Here's how the part is built. I have some questions about the finished solid (model axes, mm). A direction names the side the tool comes from. Round coordinates to 2 decimals unless told otherwise and drop trailing zeros. Loops run counter-clockwise (first coordinate to the right, second up) from the corner with the lowest first, then second, coordinate; pieces in that order, holes last. Notation, with made-up numbers: M 12.5,5.5 L 67.5,5.5 A23 cw 67.5,27.5 Z; hole C 70,-23.75 d1. An arc over 180 degrees is marked long. Write each question's results on one line, items separated by ' | '. Start each with the question number.
```python
from build123d import *

# Parameters (mm, degrees)
SKETCH_1_W          = 15
SKETCH_1_H          = 26
SKETCH_1_R          = 2.5
SKETCH_1_R_2        = 1.5
EXTRUDE_1_DEPTH     = 4
SKETCH_14_W         = 15
SKETCH_14_H         = 6
EXTRUDE_4_DEPTH     = 20
EXTRUDE_5_DEPTH     = 4
SKETCH_17_W         = 40
SKETCH_17_H         = 10
CUT_EXTRUDE_3_DEPTH = 1.5
SKETCH_18_R         = 1.5
CUT_EXTRUDE_4_DEPTH = 2.5
CUT_EXTRUDE_5_DEPTH = 1.5
SKETCH_20_R         = 1.5
CUT_EXTRUDE_6_DEPTH = 2.5
FILLET_1_R          = 2
FILLET_2_R          = 1


with BuildPart() as part:
    # 草图1 → 凸台-拉伸1 (new body)
    with BuildSketch(Plane.XY):
        with Locations((0, -3)):
            Rectangle(SKETCH_1_W, SKETCH_1_H)
        Circle(SKETCH_1_R, mode=Mode.SUBTRACT)
        with Locations((-4, 6)):
            Circle(SKETCH_1_R_2, mode=Mode.SUBTRACT)
        with Locations((4, -6)):
            Circle(SKETCH_1_R_2, mode=Mode.SUBTRACT)
    extrude(amount=EXTRUDE_1_DEPTH)

    # 草图14 → 凸台-拉伸4 (add)
    with BuildSketch(Plane.XY.offset(4)):
        with Locations((0, -13)):
            Rectangle(SKETCH_14_W, SKETCH_14_H)
    extrude(amount=EXTRUDE_4_DEPTH)

    # 草图15 → 凸台-拉伸5 (add)
    with BuildSketch(Plane.XY.offset(24)):
        Polygon((-7.5, -10), (-7.5, -39.01879788), (-26.52, -50), (-77.5, -50), (-77.5, -65), (-22.5, -65), (7.5, -47.679491924), (7.5, -10), align=None)
    extrude(amount=EXTRUDE_5_DEPTH)

    # 草图17 → 切除-拉伸3 (cut)
    with BuildSketch(Plane(origin=(0, 0, 24), x_dir=(-1, 0, 0), z_dir=(0, 0, -1))):
        with Locations((54.5, -57.5)):
            Rectangle(SKETCH_17_W, SKETCH_17_H)
    extrude(amount=-CUT_EXTRUDE_3_DEPTH, mode=Mode.SUBTRACT)

    # 草图18 → 切除-拉伸4 (cut)
    with BuildSketch(Plane(origin=(0, 0, 25.5), x_dir=(-1, 0, 0), z_dir=(0, 0, -1))):
        with Locations((39.5, -57.5)):
            Circle(SKETCH_18_R)
        with Locations((49.5, -57.5)):
            Circle(SKETCH_18_R)
        with Locations((59.5, -57.5)):
            Circle(SKETCH_18_R)
        with Locations((69.5, -57.5)):
            Circle(SKETCH_18_R)
    extrude(amount=-CUT_EXTRUDE_4_DEPTH, mode=Mode.SUBTRACT)

    # 草图19 → 切除-拉伸5 (cut)
    with BuildSketch(Plane(origin=(0, 0, 24), x_dir=(-1, 0, 0), z_dir=(0, 0, -1))):
        Polygon((6.699491924, -41.443375673), (24.02, -51.443375673), (19.02, -60.103629711), (1.699491924, -50.103629711), align=None)
    extrude(amount=-CUT_EXTRUDE_5_DEPTH, mode=Mode.SUBTRACT)

    # 草图20 → 切除-拉伸6 (cut)
    with BuildSketch(Plane(origin=(0, 0, 25.5), x_dir=(-1, 0, 0), z_dir=(0, 0, -1))):
        with Locations((8.529618943, -48.273502692)):
            Circle(SKETCH_20_R)
        with Locations((17.189872981, -53.273502692)):
            Circle(SKETCH_20_R)
    extrude(amount=-CUT_EXTRUDE_6_DEPTH, mode=Mode.SUBTRACT)

    # 圆角1
    fillet_1_edges = [part.edges().sort_by_distance(p)[0] for p in [
        (-7.5, 0, 4),
        (7.5, 0, 4),
        (-7.5, -10, 16),
        (0, -10, 4),
        (7.5, -10, 16),
        (0, -16, 24),
        (-77.5, -50, 26),
        (-77.5, -65, 26),
        (0, -10, 28),
        (-7.5, -24.50939894, 28),
        (-17.01, -44.50939894, 28),
        (-52.01, -50, 28),
        (-77.5, -57.5, 28),
        (-50, -65, 28),
        (7.5, -28.839745962, 28),
        (0, -16, 0),
    ]]
    fillet(fillet_1_edges, radius=FILLET_1_R - 0.0001)  # a hair under: the kernel refuses the full size

    # 圆角2
    fillet_2_edges = [part.edges().sort_by_distance(p)[0] for p in [
        (7.5, 10, 1.00005),
        (-7.5, 10, 1.00005),
        (0, 10, 4),
        (-6.914242852, 10, 3.414242852),
        (6.914242852, 10, 3.414242852),
    ]]
    fillet(fillet_2_edges, radius=FILLET_2_R)


solid = part.part
```
1. I want a section at D-D on z = 15.25. List the corners of the cut face in (x, y) for me, plus the area to 3 significant figures.
2. I need wall thicknesses on line 1 along Y through (x, z) = (0, 2.1); line 2 along Y through (x, z) = (4, 1.9); line 3 along Z through (x, y) = (-3, -51.5). Which ranges of each line are inside material? Lowest first, please.
3. Which directions (+Z, -Z, +X, -X, +Y, -Y) give clear straight access to the entire face, cutting with the end or side of a thin tool? Please do faces 4 (the face through (-19, -48, 24)), 5 (the face through (-21.555, -55.713, 24.74)), 6 (the face through (-51, -50, 25)), 7 (the face through (0, 3, 4)).
4. If we mould it in two halves opening along X, with no side actions, what happens to faces 1 (the face through (-15.69, -53.21, 26.73)), 2 (the face through (6.9, -10.57, 15.86)), 3 (the face through (-46.87, -64.4, 27.43))? For each: released by +X, released by -X, zero draft, split by the parting line, or undercut.
5. I want a section at B-B on x = -59.5. List the corners of the cut face in (y, z) for me.
6. I want a section at C-C on x = -45.5. List the corners of the cut face in (y, z) for me, plus the area to 3 significant figures.
7. For pin 1 (5 mm diameter, centred on x = -64, y = -48.5, fed in from -Z); pin 2 (4 mm diameter, centred on x = -69.5, y = -57.5, fed in from -Z); pin 3 (3.5 mm diameter, centred on x = -2.5, y = -3, fed in from +Z), each with a flat end and sliding along its axis, tell me the tip position at first contact or that it passes through.
Outcome:
1) outline: M -7.5,-16 L 7.5,-16 L 7.5,-12 A2 ccw 5.5,-10 L -5.5,-10 A2 ccw -7.5,-12 Z | area: 88.3 mm2
2) line 1: -16 to -2.5, 2.5 to 10 | line 2: -16 to -7.5, -4.5 to 10 | line 3: 24 to 28
3) face 4: -Z, +X, -X, -Y | face 5: -Z | face 6: +Z, -Z, -X, +Y | face 7: +Z, +X, -X, +Y
4) face 1: undercut | face 2: released by +X | face 3: zero draft
5) outline: M -65,24 L -62.5,24 L -62.5,25.5 L -59,25.5 L -59,28 L -63,28 A2 ccw -65,26 Z; M -56,25.5 L -52.5,25.5 L -52.5,24 L -50,24 L -50,26 A2 ccw -52,28 L -56,28 Z
6) outline: M -65,24 L -62.5,24 L -62.5,25.5 L -52.5,25.5 L -52.5,24 L -50,24 L -50,26 A2 ccw -52,28 L -63,28 A2 ccw -65,26 Z | area: 43.3 mm2
7) pin 1: z = 24 | pin 2: z = 25.5 | pin 3: z = 4
